from build123d import *

# Parameters (mm, degrees)
SKETCH1_R          = 7.5
EXTRUDE1_DEPTH     = 43
SKETCH2_R          = 4
EXTRUDE2_DEPTH     = 14
CUT_EXTRUDE1_START = -7
CUT_EXTRUDE1_DEPTH = 7
CHAMFER1_SIZE      = 0.5


with BuildPart() as part:
    # Sketch1 → Extrude1 (new body)
    with BuildSketch(Plane(origin=(0, 0, 0), x_dir=(1, 0, 0), z_dir=(0, 1, 0))):
        with Locations(Location((0, 0, 0), (0, 0, 270))):
            Circle(SKETCH1_R)
    extrude(amount=EXTRUDE1_DEPTH)

    # Sketch2 → Extrude2 (add)
    with BuildSketch(Plane.XZ):
        with Locations(Location((0, 0, 0), (0, 0, 90))):
            Circle(SKETCH2_R)
    extrude(amount=EXTRUDE2_DEPTH)

    # Sketch4 → Cut-Extrude1 (cut)
    with BuildSketch(Plane(origin=(0, 43, 0), x_dir=(-1, 0, 0), z_dir=(0, 1, 0)).offset(CUT_EXTRUDE1_START)):
        with BuildLine():
            Line((-5, -5.590169944), (-5, 5.590169944))
            ThreePointArc((-5, 5.590169944), (-7.5, 0), (-5, -5.590169944))
        make_face()
        with BuildLine():
            ThreePointArc((7.5, 0), (6.846531969, 3.061862178), (5, 5.590169944))
            Line((5, 5.590169944), (5, -5.590169944))
            ThreePointArc((5, -5.590169944), (6.846531969, -3.061862178), (7.5, 0))
        make_face()
    extrude(amount=CUT_EXTRUDE1_DEPTH, mode=Mode.SUBTRACT)

    # Chamfer1
    chamfer1_edges = [part.edges().sort_by_distance(p)[0] for p in [
        (0, 0, -7.5),
        (0, -14, -4),
    ]]
    chamfer(chamfer1_edges, length=CHAMFER1_SIZE)

    # Sketch5 → Cut-Revolve2 (revolve, cut)
    with BuildSketch(Plane.XY, mode=Mode.PRIVATE) as cut_revolve2_sk:
        Polygon((0, 43), (4.2, 43), (4.2, 25), (0, 22.4763854), align=None)
    revolve(cut_revolve2_sk.sketch.rotate(Axis((0, 0, 0), (0, 1, 0)), 131.810314896), axis=Axis((0, 0, 0), (0, 1, 0)), mode=Mode.SUBTRACT)


solid = part.part
Can you work these out from the model? Positions are in its coordinate system, mm. A direction names the side the tool comes from. Give positions to 0.01 mm unless a question says otherwise; leave off trailing zeros. Write each loop counter-clockwise with the first axis right and the second up, starting at its lowest first coordinate (ties: lowest second). Pieces come first, ordered by that corner, then holes. Notation, with made-up numbers: (72, 21) -> (98, 21) arc R20 ccw to (98, 45) -> close; hole circle Ø3 at (14.25, 11.5). An arc over 180 degrees is marked (long way). Answer as a JSON object with one key per item and string values. Group by question number.
Item 1: Please list where these lines run through material, in increasing order: line 1 (X direction, y = 30, z = 0); line 2 (Y direction, x = 3.25, z = -4). Write a range as [from, to].
Item 2: For faces 1 (the face through (5, 39, 0)), 2 (the face through (4.127, 33.874, 0.78)), 3 (the face through (-6, 36, 0)), 4 (the face through (3.905, -6.656, -0.867)), which set-ups out of +Z, -Z, +X, -X, +Y, -Y let a thin tool reach every point of the face, with its end or its side?
Item 3: I'm going to push flat-ended pins straight in: P1, Ø2, axis at x = -1.5, y = 23.5, coming from the +Z side; P2, Ø0.8, axis at x = -6.5, z = 1.5, coming from the +Y side; P3, Ø2, axis at x = 2, y = 12.5, coming from the -Z side. Where does each tip first touch, or does it pass through?
Item 4: Suppose I cut it at A-A (y = 11). Please give me the cut outline in (x, z), plus the area to 3 significant figures.
Item 5: We'd pull the mould along X, two halves only. Please class faces 5 (the face through (-0.58, 22.88, -0.34)), 6 (the face through (-5, 39, 0)), 7 (the face through (6, 36, 0)): +X half, -X half, draft (parallel to the pull), parting line (faces both ways), or undercut.
Findings:
{
 "1": {"line 1": "x = [-7.5, -4.2], [4.2, 7.5]", "line 2": "y = [0, 43]"},
 "2": {"face 1": "+Z, -Z, +X, +Y", "face 2": "+Y", "face 3": "+Z, -Z, -X, +Y", "face 4": "-Y"},
 "3": {"P1": "stops at z = 7.48", "P2": "stops at y = 36", "P3": "stops at z = -7.43"},
 "4": {"outline": "circle Ø15 at (0, 0)", "area": "177 mm²"},
 "5": {"face 5": "undercut", "face 6": "-X half", "face 7": "draft"}
}
